from build123d import *

# Parameters (mm, degrees)
F1_DEPTH = 4.7625
F3_D     = 6.35


with BuildPart() as f1:
    # F0 (on Front) → F1 (new body, symmetric)
    with BuildSketch(Plane.XZ):
        with BuildLine():
            ThreePointArc((107.490789, -0.614724), (0, 107.492547), (-107.490789, -0.614724))
            Line((-107.490789, -0.614724), (107.490789, -0.614724))
        make_face()
    extrude(amount=F1_DEPTH, both=True)

    # F3 (through all)
    with Locations(Plane.XZ.offset(4.7625)):
        with Locations((23.8125, 18.435276), (87.3125, 18.661174), (47.904196, 77.188074), (23.586602, 81.935276), (68.554047, 63.49629), (82.392403, 42.944376), (-23.8125, 18.435276), (-23.586602, 81.935276), (-47.904196, 77.188074), (-68.554047, 63.49629), (-82.392403, 42.944376), (-87.3125, 18.661174)):
            Hole(F3_D / 2)


solid = f1.part
Geometry: final body of the model. Coordinates: model frame, mm. Coordinates: 2 decimals unless noted, no trailing zeros. Order: outer loops, then holes, each group sorted by start corner. A loop starts at its lowest first (then second) coordinate and runs counter-clockwise, first axis right, second up.
1) First-contact query: P1, Ø8.5, axis at x = -47.9, z = 77.19, coming from the -Y side; P2, Ø1, axis at y = -1, z = 85.5, coming from the +X side; P3, Ø3, axis at y = -1.5, z = 50.5, coming from the +X side; P4, Ø4, axis at y = 1, z = 70, coming from the +X side. Flat tips, straight axial feed; report the tip coordinate or a pass-through.
Result sheet:
P1: stops at y = -4.76
P2: stops at x = 65.8
P3: stops at x = 95.67
P4: stops at x = 83.25
2) Section B-B (z = 94). Return loops of the section in (x, y).
Result sheet:
outline: (-52.14, -4.76) - (52.14, -4.76) - (52.14, 4.76) - (-52.14, 4.76) - close
3) Section C-C (x = 60). Return loops of the section in (y, z), then the cut area to 3 significant figures.
Result sheet:
outline: (-4.76, -0.61) - (4.76, -0.61) - (4.76, 89.19) - (-4.76, 89.19) - close
area: 855 mm2
4) Ray query, probe 1 along Z at (x, y) = (23, -0.75); probe 2 along X at (y, z) = (-2.25, 77.5); probe 3 along X at (y, z) = (0.5, 21). Return the intervals inside material, ascending.
Result sheet:
probe 1: z = -0.61 to 15.37, 21.5 to 78.81, 85.06 to 105
probe 2: x = -74.49 to -51.06, -44.74 to 44.74, 51.06 to 74.49
probe 3: x = -105.42 to -89.46, -85.17 to -25.68, -21.94 to 21.94, 25.68 to 85.17, 89.46 to 105.42
5) Section A-A (y = 3.25). Give the number of separate pieces and of enclosed holes in the cut face, then the cut area to 3 significant figures.
Result sheet:
separate pieces: 1
enclosed holes: 12
area: 17,900 mm2
